The figure shows three views and two pictorial views of one solid part (mm, origin at its lowest corner). Answer the questions. A direction names the side the tool comes from. Give positions to 0.01 mm unless a question says otherwise; leave off trailing zeros. Loops run counter-clockwise (first coordinate to the right, second up) from the corner with the lowest first, then second, coordinate; pieces in that order, holes last. Notation, with made-up numbers: (60.25, 21) - (77.25, 21) arc R25 ccw to (77.25, 47) - close; hole circle Ø5 at (58, 53). An arc over 180 degrees is marked (long way). Use a Markdown table: item, result. Add a question column.
Item 1: Consider probe 1 along X at (y, z) = (0.75, 8.25); probe 2 along Z at (x, y) = (2.54, 3.6); probe 3 along X at (y, z) = (4.25, 6.25). Determine where each line is inside the solid, lowest interval first. Write a range as [from, to].
Item 2: A cutting plane is placed at B-B (x = 5). Determine the outline of the cut face in (y, z).
Item 3: Which of the six approach directions +Z, -Z, +X, -X, +Y, -Y give full straight-line access (tool end or side, diameter ignored) to the marked faces 4, 5, 6, 7 and 8?
Item 4: For a pull along Z with two mould halves and no side action, classify the marked faces 1, 2 and 3 as +Z half, -Z half, draft (parallel to the pull), parting line (faces both ways), or undercut.
Item 5: Each of these flat-tipped pins is pushed along its axis until it touches: P1, Ø3, axis at x = 3, z = 6, coming from the -Y side; P2, Ø0.8, axis at x = 7, y = 0.5, coming from the +Z side (1 decimal); P3, Ø1.4, axis at x = 2, z = 6.5, coming from the -Y side. Where does it stop, or does it pass through?
Item 6: A cutting plane is placed at A-A (z = 8.5). Determine the outline of the cut face in (x, y), plus the area to 3 significant figures.
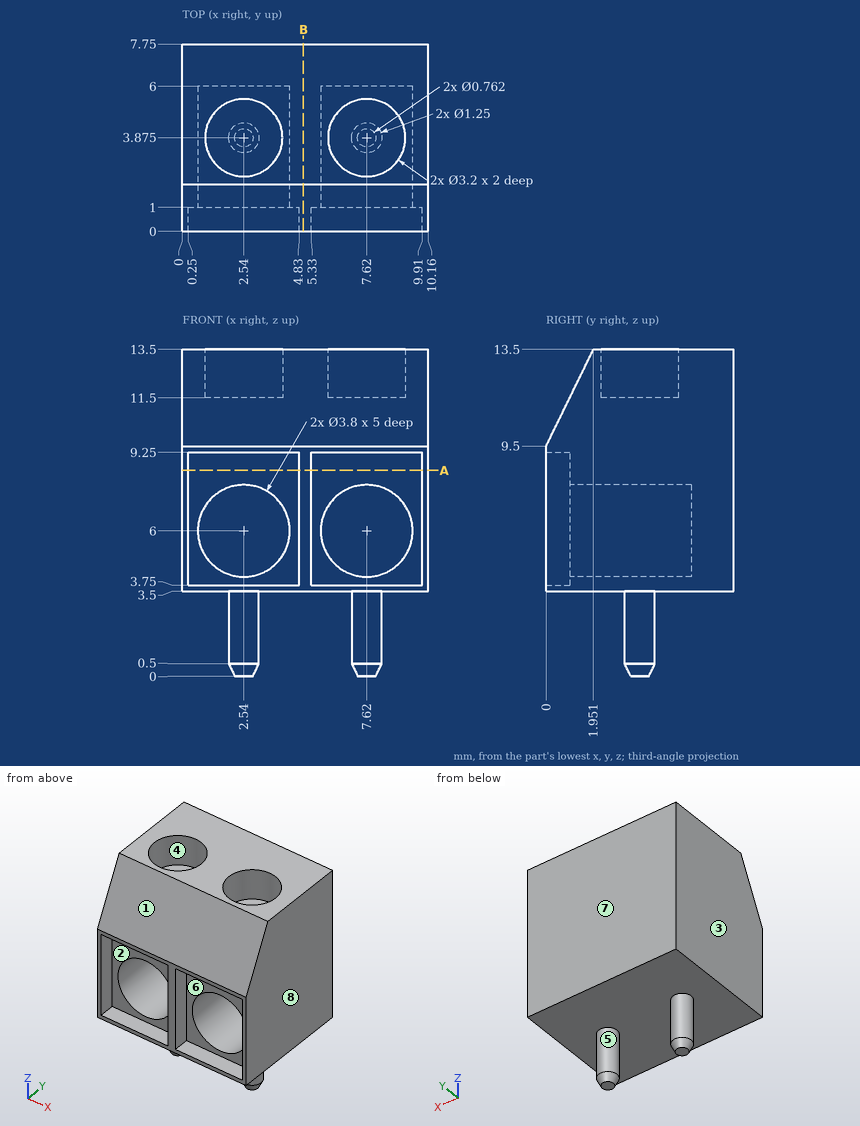
Geometry says:
| question | item | result |
|---|---|---|
| 1 | probe 1 | [0, 0.25], [4.83, 5.33], [9.91, 10.16] |
| 1 | probe 2 | [0, 4.1], [7.9, 11.5] |
| 1 | probe 3 | [0, 0.66], [4.42, 5.74], [9.5, 10.16] |
| 2 | outline | (0, 3.5) - (7.75, 3.5) - (7.75, 13.5) - (1.95, 13.5) - (0, 9.5) - close |
| 3 | face 4 | +Z |
| 3 | face 5 | -Z |
| 3 | face 6 | -Y |
| 3 | face 7 | +Z, -Z, +X, -X, +Y |
| 3 | face 8 | +Z, -Z, +X, +Y, -Y |
| 4 | face 1 | +Z half |
| 4 | face 2 | undercut |
| 4 | face 3 | draft |
| 5 | P1 | y = 1 |
| 5 | P2 | z = 11.3 |
| 5 | P3 | y = 6 |
| 6 | outline | (0, 0) - (0.25, 0) - (0.25, 1) - (4.83, 1) - (4.83, 0) - (5.33, 0) - (5.33, 1) - (9.91, 1) - (9.91, 0) - (10.16, 0) - (10.16, 7.75) - (0, 7.75) - close |
| 6 | area | 69.6 mm² |
